```python
from build123d import *

# Parameters (mm, degrees)
F0_W      = 140
F0_H      = 140
F1_DEPTH  = 40
F4_DEPTH  = 145
F5_DEPTH  = 145
F6_DEPTH  = 5
F7_DEPTH  = 5
F2_W      = 5
F2_H      = 40
F8_DEPTH  = 5
F9_DEPTH  = 5
F10_W     = 10
F10_H     = 10
F11_DEPTH = 3.5
F10_W_2   = 20
F10_H_2   = 20
F12_DEPTH = 5


with BuildPart() as f1:
    # F0 (on Top) → F1 (new body, symmetric)
    with BuildSketch(Plane.XY):
        Rectangle(F0_W, F0_H)
    extrude(amount=F1_DEPTH, both=True)

    # F3 (on face) → F4 (join)
    with BuildSketch(Plane(origin=(-70, 0, 0), x_dir=(0, -1, 0), z_dir=(-1, 0, 0))):
        Polygon((-70, -40), (70, -40), (70, 0), (53.6, 0), (53.6, -10), (32.2, -10), (32.2, 0), (10.8, 0), (10.8, -10), (-10.8, -10), (-10.8, 0), (-32.2, 0), (-32.2, -10), (-53.6, -10), (-53.6, 0), (-70, 0), align=None)
    extrude(amount=-F4_DEPTH)

    # F2 (on face) → F5 (join)
    with BuildSketch(Plane(origin=(0, 70, 0), x_dir=(-1, 0, 0), z_dir=(0, 1, 0))):
        Polygon((-70, -40), (70, -40), (70, 0), (53.6, 0), (53.6, -10), (32.2, -10), (32.2, 0), (10.8, 0), (10.8, -10), (-10.8, -10), (-10.8, 0), (-32.2, 0), (-32.2, -10), (-53.6, -10), (-53.6, 0), (-70, 0), align=None)
    extrude(amount=-F5_DEPTH)

    # F2 (on face) → F6 (join)
    with BuildSketch(Plane(origin=(0, 70, 0), x_dir=(-1, 0, 0), z_dir=(0, 1, 0))):
        Polygon((-70, -40), (70, -40), (70, 0), (53.6, 0), (53.6, -10), (32.2, -10), (32.2, 0), (10.8, 0), (10.8, -10), (-10.8, -10), (-10.8, 0), (-32.2, 0), (-32.2, -10), (-53.6, -10), (-53.6, 0), (-70, 0), align=None)
    extrude(amount=F6_DEPTH)

    # F3 (on face) → F7 (join)
    with BuildSketch(Plane(origin=(-70, 0, 0), x_dir=(0, -1, 0), z_dir=(-1, 0, 0))):
        Polygon((-70, -40), (70, -40), (70, 0), (53.6, 0), (53.6, -10), (32.2, -10), (32.2, 0), (10.8, 0), (10.8, -10), (-10.8, -10), (-10.8, 0), (-32.2, 0), (-32.2, -10), (-53.6, -10), (-53.6, 0), (-70, 0), align=None)
    extrude(amount=F7_DEPTH)

    # F2 (on face) → F8 (join, through all)
    with BuildSketch(Plane(origin=(0, 70, 0), x_dir=(-1, 0, 0), z_dir=(0, 1, 0))):
        with Locations((-72.5, -20)):
            Rectangle(F2_W, F2_H)
        with Locations((72.5, -20)):
            Rectangle(F2_W, F2_H)
    extrude(amount=F8_DEPTH)

    # F9 (add, through all): faces of the model
    f9_faces = [f1.faces().sort_by_distance(p)[0] for p in [
        (72.5, -70, -20),
        (-72.5, -70, -20),
    ]]
    extrude(f9_faces, amount=F9_DEPTH)

    # F10 (on face) → F11 (join)
    with BuildSketch(Plane(origin=(0, 0, -40), x_dir=(1, 0, 0), z_dir=(0, 0, -1))):
        with Locations((-55, 5)):
            Rectangle(F10_W, F10_H)
        with Locations((-35, -15)):
            Rectangle(F10_W, F10_H)
        with Locations((-45, -55)):
            Rectangle(F10_W, F10_H)
        with Locations((25, 15)):
            Rectangle(F10_W, F10_H)
        with Locations((15, 35)):
            Rectangle(F10_W, F10_H)
        with Locations((45, 55)):
            Rectangle(F10_W, F10_H)
    extrude(amount=F11_DEPTH)

    # F10 (on face) → F12 (join)
    with BuildSketch(Plane(origin=(0, 0, -40), x_dir=(1, 0, 0), z_dir=(0, 0, -1))):
        with Locations((40, -10)):
            Rectangle(F10_W_2, F10_H_2)
        Rectangle(F10_W_2, F10_H_2)
        with Locations((-40, 30)):
            Rectangle(F10_W_2, F10_H_2)
        with Locations((10, -40)):
            Rectangle(F10_W_2, F10_H_2)
    extrude(amount=F12_DEPTH)


solid = f1.part
```
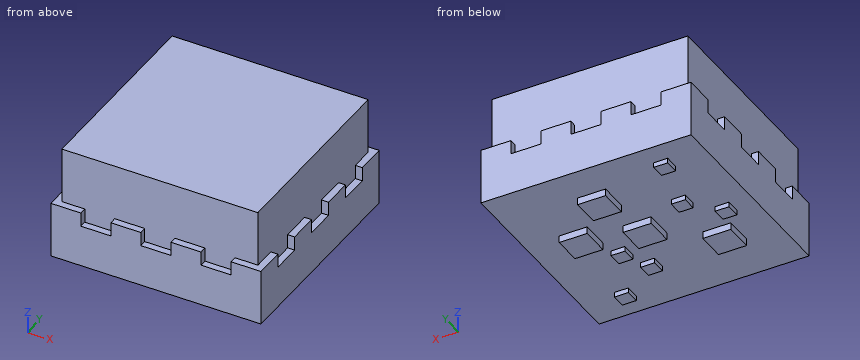
Verification items for the finished model (mm, model axes). Coordinates: 2 decimals unless noted, no trailing zeros. Write each loop counter-clockwise with the first axis right and the second up, starting at its lowest first coordinate (ties: lowest second). Pieces come first, ordered by that corner, then holes. Notation, with made-up numbers: M 18,61 L 27,61 A17 cw 27,78 Z; hole C 63.5,-15 d9. An arc over 180 degrees is marked long. One line per item, written item: value.
Item 1: Section check D-D, the plane z = 27.5. Record the boundary of the cut face in (x, y).
Check sheet entries:
outline: M -70,-70 L 70,-70 L 70,70 L -70,70 Z
Item 2: Gauge pin test, flat ends, axial feed: pin 1 Ø5.5 at (x, y) = (-21, 73) entering from +Z; pin 2 Ø1.5 at (y, z) = (-46.5, -1.5) entering from -X; pin 3 Ø8 at (y, z) = (52, -8) entering from -X; pin 4 Ø1.5 at (x, z) = (0.5, -42.5) entering from -Y. Record the tip position at first contact, or that the pin passes through.
Check sheet entries:
pin 1: stops at z = 0
pin 2: stops at x = -70
pin 3: stops at x = -75
pin 4: stops at y = -10
Item 3: Section check C-C, the plane x = 17. Record the boundary of the cut face in (y, z), plus the area to 3 significant figures.
Check sheet entries:
outline: M -75,-40 L -40,-40 L -40,-43.5 L -30,-43.5 L -30,-40 L 30,-40 L 30,-45 L 50,-45 L 50,-40 L 75,-40 L 75,0 L 70,0 L 70,40 L -70,40 L -70,0 L -75,0 Z
area: 11,700 mm^2
Item 4: Scan lines: line 1 along Z through (x, y) = (-33.5, 6); line 2 along Y through (x, z) = (-21, 36.5). Record each from-to range of solid material in increasing order.
Check sheet entries:
line 1: z = -40 to 40
line 2: y = -70 to 70
Item 5: Section check B-B, the plane y = -57.5. Record the boundary of the cut face in (x, z).
Check sheet entries:
outline: M -75,-40 L 40,-40 L 40,-43.5 L 50,-43.5 L 50,-40 L 75,-40 L 75,0 L 70,0 L 70,40 L -70,40 L -70,0 L -75,0 Z
Item 6: Section check A-A, the plane x = 45.5. Record the boundary of the cut face in (y, z), plus the area to 3 significant figures.
Check sheet entries:
outline: M -75,-40 L -60,-40 L -60,-43.5 L -50,-43.5 L -50,-40 L 0,-40 L 0,-45 L 20,-45 L 20,-40 L 75,-40 L 75,-10 L 70,-10 L 70,40 L -70,40 L -70,-10 L -75,-10 Z
area: 11,600 mm^2
